Source: three-view drawing plus pictorial views. Frame: mm from the lowest corner of the part. A direction names the side the tool comes from. Give positions to 0.01 mm unless a question says otherwise; leave off trailing zeros. Write each loop counter-clockwise with the first axis right and the second up, starting at its lowest first coordinate (ties: lowest second). Pieces come first, ordered by that corner, then holes. Notation, with made-up numbers: (-30, 2.25) -> (6, 2.25) arc R11 cw to (6, 15.25) -> close; hole circle Ø1 at (82, 74). An arc over 180 degrees is marked (long way). Answer in a Markdown table with one row per item. Add a question column.
Item 1: Material intervals for probe 1 along Z at (x, y) = (1.5, 6.5); probe 2 along Z at (x, y) = (9, 5.5); probe 3 along X at (y, z) = (1.25, 21), sorted ascending. Write a range as from..to.
Item 2: First-contact query: P1, Ø9, axis at x = 8.5, z = 3.5, coming from the -Y side; P2, Ø3.5, axis at y = 4, z = 27, coming from the -X side; P3, Ø5, axis at x = 7.5, z = 12.5, coming from the +Y side. Flat tips, straight axial feed; report the tip coordinate or a pass-through.
Item 3: Access query for the marked faces 3 and 4. Directions: +Z, -Z, +X, -X, +Y, -Y. A direction counts if a zero-diameter tool reaches every point of the face in a straight line with its end or side. Return the directions, or none.
Item 4: Section query D-D on y = 1.5. Output: boundary loops of the cut face in (x, z), plus the area to 3 significant figures.
Item 5: Section query A-A on z = 39.5. Output: boundary loops of the cut face in (x, y), plus the area to 3 significant figures.
Item 6: Section query C-C on y = 6. Output: boundary loops of the cut face in (x, z).
Item 7: Draft query along Z for the marked faces 1 and 2. Return one class per face: +Z half, -Z half, draft (parallel to the pull), parting line (faces both ways), or undercut.
Item 8: Section query B-B on x = 26. Output: boundary loops of the cut face in (y, z), plus the area to 3 significant figures.
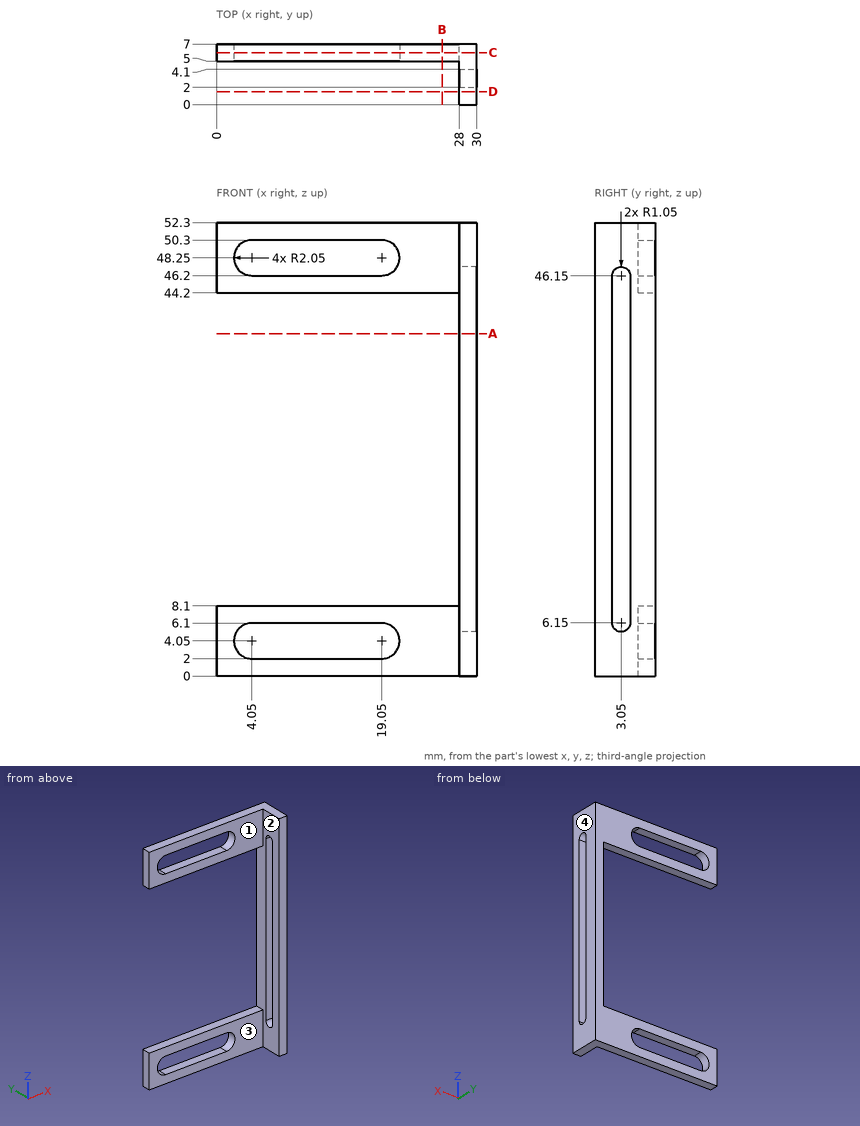
Findings below:
| question | item | result |
|---|---|---|
| 1 | probe 1 | z = 0..8.1, 44.2..52.3 |
| 1 | probe 2 | z = 0..2, 6.1..8.1, 44.2..46.2, 50.3..52.3 |
| 1 | probe 3 | x = 28..30 |
| 2 | P1 | stops at y = 5 |
| 2 | P2 | stops at x = 28 |
| 2 | P3 | passes through |
| 3 | face 3 | +Z, -Z, -X, -Y |
| 3 | face 4 | +Z, -Z, +X, +Y, -Y |
| 4 | outline | (28, 0) -> (30, 0) -> (30, 52.3) -> (28, 52.3) -> close |
| 4 | area | 105 mm^2 |
| 5 | outline | (28, 0) -> (30, 0) -> (30, 2) -> (28, 2) -> close; (28, 4.1) -> (30, 4.1) -> (30, 7) -> (28, 7) -> close |
| 5 | area | 9.80 mm^2 |
| 6 | outline | (0, 0) -> (30, 0) -> (30, 52.3) -> (0, 52.3) -> (0, 44.2) -> (28, 44.2) -> (28, 8.1) -> (0, 8.1) -> close; hole (4.05, 2) -> (19.05, 2) arc R2.05 ccw to (19.05, 6.1) -> (4.05, 6.1) arc R2.05 ccw to start; hole (4.05, 46.2) -> (19.05, 46.2) arc R2.05 ccw to (19.05, 50.3) -> (4.05, 50.3) arc R2.05 ccw to start |
| 7 | face 1 | draft |
| 7 | face 2 | undercut |
| 8 | outline | (5, 0) -> (7, 0) -> (7, 8.1) -> (5, 8.1) -> close; (5, 44.2) -> (7, 44.2) -> (7, 52.3) -> (5, 52.3) -> close |
| 8 | area | 32.4 mm^2 |
